Read the model definition and answer for the solid it produces. Units are mm, in the model's axes. Coordinates: 2 decimals unless noted, no trailing zeros. Write each loop counter-clockwise with the first axis right and the second up, starting at its lowest first coordinate (ties: lowest second). Pieces come first, ordered by that corner, then holes. Notation, with made-up numbers: (21, 0) -> (40, 0) arc R18 cw to (40, 16) -> close; hole circle Ø1 at (38, -11). An arc over 180 degrees is marked (long way). Use CSV: the item, a comma, the result in double quotes.
from build123d import *

# Parameters (mm, degrees)
F0_W        = 38.1
F0_H        = 2.54
F1_DEPTH    = 8.255
F3_R        = 1.778
F4_T1_DEPTH = 47.2449047052
F5_DEPTH    = 25.4


# Not quite as in the source:
# - a fillet or chamfer that OpenCascade refuses, or shapes differently, is made with other operations: its cross-section is extruded or revolved along the edge and cut away or added


with BuildPart() as f1:
    # F0 (on Top) → F1 (new body)
    with BuildSketch(Plane.XY):
        with Locations((0, 1.27)):
            Rectangle(F0_W, F0_H)
    extrude(amount=F1_DEPTH)

    # F3
    f3_edges = [f1.edges().sort_by_distance(p)[0] for p in [
        (0, 2.54, 8.255),
    ]]
    fillet(f3_edges, radius=F3_R)

    # F4: chamfer of 1.778 on 1 edges, made by hand

    # F4_s2 → F4_t1 (cut)
    with BuildSketch(Plane.YZ.offset(-23.6224523526)):
        Polygon((1.778, 8.255), (0, 6.477), (0, 8.255), align=None)
    extrude(amount=F4_T1_DEPTH, mode=Mode.SUBTRACT)

    # F2 (on face) → F5 (cut)
    with BuildSketch(Plane.XZ):
        Polygon((-16.51, 6.6902954744), (-15.6066174209, 8.255), (-17.4133825791, 8.255), align=None)
        Polygon((-4.6817409051, 8.255), (-6.3418590949, 8.255), (-5.5118, 6.8172954744), align=None)
        Polygon((6.4885060633, 8.255), (4.5350939367, 8.255), (5.5118, 6.5632954744), align=None)
        Polygon((17.3400590949, 8.255), (15.6799409051, 8.255), (16.51, 6.8172954744), align=None)
    extrude(amount=-F5_DEPTH, mode=Mode.SUBTRACT)


solid = f1.part
1. This flat-tipped pin is pushed along its axis until it touches: pin 1 Ø1 at (x, y) = (-8.5, 1) entering from -Z. Where does it stop, or does it pass through?
Solutions:
pin 1,"stops at z = 0"
2. Find the intervals of material crossed by line 1 along X through (y, z) = (1.95, 7.5); line 2 along Z through (x, y) = (14.5, 0.5); line 3 along Z through (x, y) = (-3.5, 1.25), in increasing order.
Solutions:
line 1,"x = -19.05 to -16.98, -16.04 to -5.91, -5.12 to 4.97, 6.05 to 16.12, 16.9 to 19.05"
line 2,"z = 0 to 6.98"
line 3,"z = 0 to 7.73"
3. For a pull along X with two mould halves and no side action, classify faces 1 (the flat face through (19.05, 1, 4)), 2 (the flat face through (16.227, 1.649, 7.308)), 3 (the flat face through (-0.267, 0.801, 7.278)), 4 (the flat face through (-19.05, 1, 4)) as pulls with the +X half, pulls with the -X half, needs draft (parallel to the pull), parting line crosses it, or undercut.
Solutions:
face 1,"pulls with the +X half"
face 2,"undercut"
face 3,"needs draft"
face 4,"pulls with the -X half"
4. A cutting plane is placed at B-B (y = 1.9). Give the vertices of the cut face in (x, z).
Solutions:
outline,"(-19.05, 0) -> (19.05, 0) -> (19.05, 7.84) -> (17.1, 7.84) -> (16.51, 6.82) -> (15.92, 7.84) -> (6.25, 7.84) -> (5.51, 6.56) -> (4.77, 7.84) -> (-4.92, 7.84) -> (-5.51, 6.82) -> (-6.1, 7.84) -> (-15.84, 7.84) -> (-16.51, 6.69) -> (-17.18, 7.84) -> (-19.05, 7.84) -> close"
5. A cutting plane is placed at A-A (x = -13). Give the vertices of the cut face in (y, z), and give its area (3 significant figures).
Solutions:
outline,"(0, 0) -> (2.54, 0) -> (2.54, 6.48) arc R1.78 ccw to (1.58, 8.06) -> (0, 6.48) -> close"
area,"18.8 mm^2"
